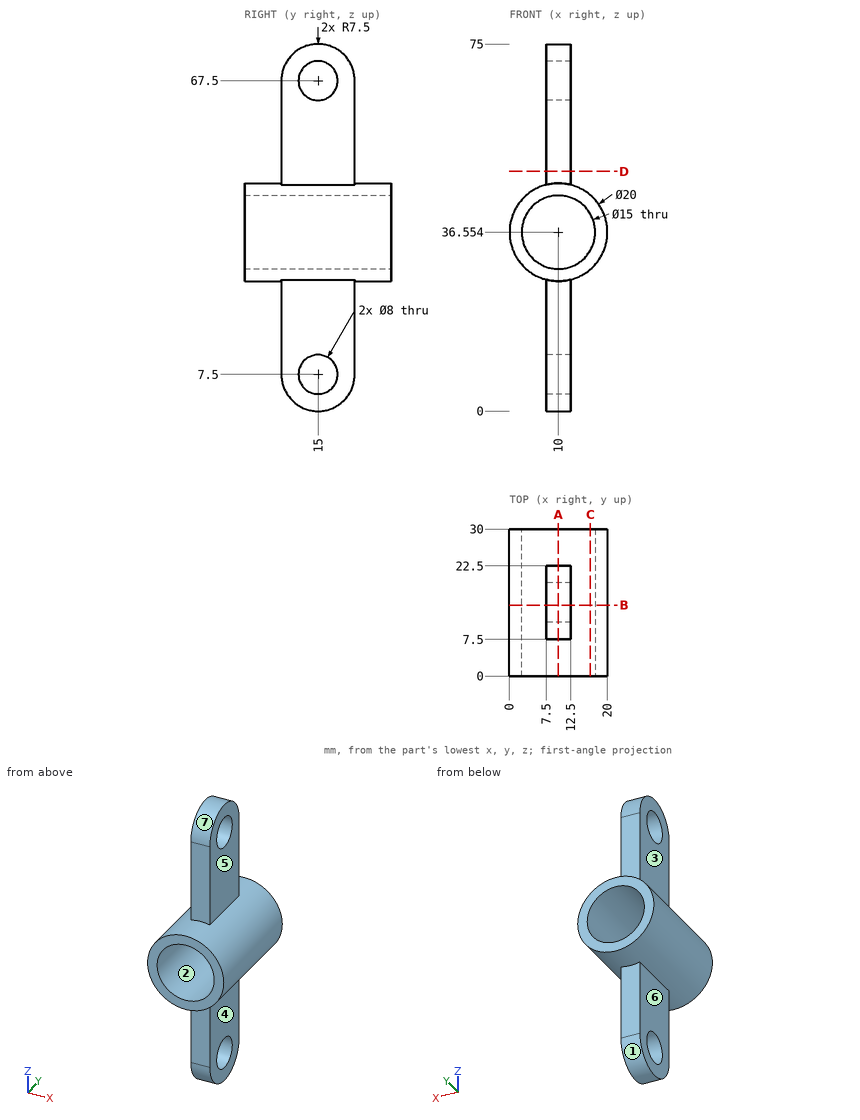
The drawing under review shows one solid part. Ordinate dimensions are in mm from its lowest x, y, z. A direction names the side the tool comes from. Coordinates: 2 decimals unless noted, no trailing zeros. Write each loop counter-clockwise with the first axis right and the second up, starting at its lowest first coordinate (ties: lowest second). Pieces come first, ordered by that corner, then holes. Notation, with made-up numbers: M -8,-23 L 17,-23 A16 ccw 17,-13 Z; hole C -35,28.25 d9. An arc over 180 degrees is marked long. Answer as a JSON object with one key per item and string values.
Item 1: Add section C-C, the plane x = 16.5. Give the boundary of the cut face in (y, z), and give its area (3 significant figures).
Outcome:
{"outline": "M 0,28.95 L 30,28.95 L 30,32.81 L 0,32.81 Z; M 0,40.3 L 30,40.3 L 30,44.15 L 0,44.15 Z", "area": "231 mm²"}
Item 2: Insertion check: pin 1 Ø12 at (y, z) = (11.5, 59) entering from +X; pin 2 Ø12 at (x, y) = (15, 3) entering from -Z; pin 3 Ø16.5 at (y, z) = (18.5, 12.5) entering from -X; pin 4 Ø7 at (y, z) = (15, 7.5) entering from +X. Each pin has a flat end and moves straight along its axis. Give the tip position at first contact, or say it passes through.
Outcome:
{"pin 1": "x = 12.5", "pin 2": "z = 3.84", "pin 3": "x = 7.5", "pin 4": "through"}
Item 3: Wall thickness on probe 1 along Z at (x, y) = (9.55, 15); probe 2 along Z at (x, y) = (10.5, 7.25); probe 3 along Z at (x, y) = (10, 12.5): over which ranges is each line inside the solid? List them lowest first.
Outcome:
{"probe 1": "0 to 3.5, 11.5 to 29.07, 44.04 to 63.5, 71.5 to 75", "probe 2": "26.57 to 29.07, 44.04 to 46.54", "probe 3": "0.43 to 4.38, 10.62 to 29.05, 44.05 to 64.38, 70.62 to 74.57"}
Item 4: Draft analysis for pull direction X (two halves, no side actions). For the marked faces 1, 2, 3 and 4, state which applies: pulls with the +X half, pulls with the -X half, needs draft (parallel to the pull), parting line crosses it, or undercut.
Outcome:
{"face 1": "needs draft", "face 2": "undercut", "face 3": "pulls with the -X half", "face 4": "pulls with the +X half"}
Item 5: Add section B-B, the plane y = 14.5. Give the boundary of the cut face in (x, z), and give its area (3 significant figures).
Outcome:
{"outline": "M 7.5,0.02 L 12.5,0.02 L 12.5,3.53 L 7.5,3.53 Z; M 7.5,11.47 L 12.5,11.47 L 12.5,26.87 A10 ccw 12.5,46.24 L 12.5,63.53 L 7.5,63.53 L 7.5,46.24 A10 ccw 7.5,26.87 Z; M 7.5,71.47 L 12.5,71.47 L 12.5,74.98 L 7.5,74.98 Z; hole C 10,36.55 d15", "area": "334 mm²"}
Item 6: Machinability: for the marked faces 5, 6 and 7, which of the approach directions +Z, -Z, +X, -X, +Y, -Y give a long, thin tool a straight path to every point of the face, cutting with its end or side? Answer none if there is none.
Outcome:
{"face 5": "+Z, +X, +Y, -Y", "face 6": "-Z, -X, +Y, -Y", "face 7": "+Z, +X, -X"}
Item 7: Add section A-A, the plane x = 10. Give the boundary of the cut face in (y, z), and give its area (3 significant figures).
Outcome:
{"outline": "M 0,26.55 L 7.5,26.55 L 7.5,7.5 A7.5 ccw 22.5,7.5 L 22.5,26.55 L 30,26.55 L 30,29.05 L 0,29.05 Z; M 0,44.05 L 30,44.05 L 30,46.55 L 22.5,46.55 L 22.5,67.5 A7.5 ccw 7.5,67.5 L 7.5,46.55 L 0,46.55 Z; hole C 15,7.5 d8; hole C 15,67.5 d8", "area": "826 mm²"}
Item 8: Add section D-D, the plane z = 49. Give the boundary of the cut face in (x, y).
Outcome:
{"outline": "M 7.5,7.5 L 12.5,7.5 L 12.5,22.5 L 7.5,22.5 Z"}
